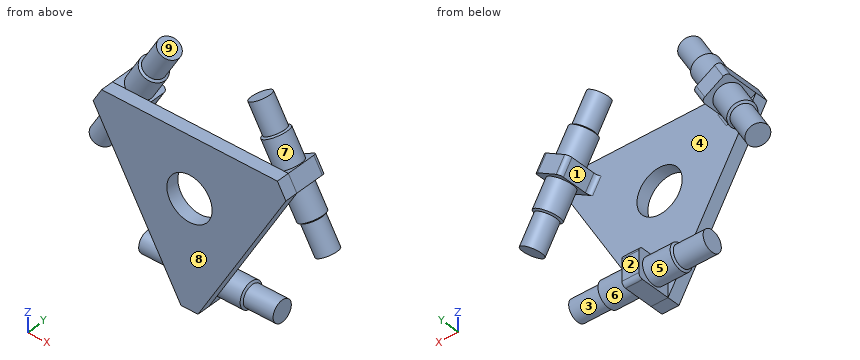
from build123d import *

# Parameters (mm, degrees)
BOSS_EXTRUDE1_DEPTH              = 3.81
F_17_32_0_53125_DIAMETER_HOLE1_D = 13.49375
BOSS_EXTRUDE2_DEPTH              = 10.16
CIRPATTERN19_COUNT               = 3
BOSS_EXTRUDE3_START              = -13.71
SKETCH6_R                        = 3.825
BOSS_EXTRUDE3_DEPTH              = 22.34
BOSS_EXTRUDE4_START              = -31.23
SKETCH7_R                        = 3.175
BOSS_EXTRUDE4_DEPTH              = 40.12
CIRPATTERN21_COUNT               = 3
CIRPATTERN28_COUNT               = 3
CHAMFER3_SIZE                    = 0.4
CHAMFER3_SIZE_2                  = 0.692820323
FILLET4_R                        = 1.27


with BuildPart() as part:
    # Sketch1 → Boss-Extrude1 (new body)
    with BuildSketch(Plane(origin=(0, 0, 0), x_dir=(1, 0, 0), z_dir=(0, 1, 0))):
        Polygon((2.54, 31.75), (-2.54, 31.75), (-28.76630657, -13.675295474), (-26.22630657, -18.074704526), (26.22630657, -18.074704526), (28.76630657, -13.675295474), align=None)
    extrude(amount=BOSS_EXTRUDE1_DEPTH)

    # 17/32 (0.53125) Diameter Hole1 (through all)
    with Locations(Plane(origin=(-6.6e-08, 3.81, -3.86e-07), x_dir=(0, 0, 1), z_dir=(0, 1, 0))):
        with Locations((0, 0)):
            Hole(F_17_32_0_53125_DIAMETER_HOLE1_D / 2)

    # Sketch5 → Boss-Extrude2 (add)
    with BuildSketch(Plane(origin=(0, 3.81, 0), x_dir=(1, 0, 0), z_dir=(0, 1, 0))):
        Polygon((-21.067340731, -9.230295474), (-28.76630657, -13.675295474), (-26.22630657, -18.074704526), (-18.527340731, -13.629704526), align=None)
    boss_extrude2 = extrude(amount=BOSS_EXTRUDE2_DEPTH)

    # CirPattern19: Boss-Extrude2 ×3 about axis
    cirpattern19_axis = Axis((0, 0, 0), (0, 1, 0))
    for i in range(1, CIRPATTERN19_COUNT):
        add(boss_extrude2.rotate(cirpattern19_axis, i * 360 / CIRPATTERN19_COUNT))

    # Sketch6 → Boss-Extrude3 (add)
    with BuildSketch(Plane(origin=(1.27, 0, 2.199704526), x_dir=(0.8660254037844383, 0, -0.5000000000000007), z_dir=(0.5000000000000007, 0, 0.8660254037844383)).offset(BOSS_EXTRUDE3_START)):
        with Locations((-27.305, 8.89)):
            Circle(SKETCH6_R)
    boss_extrude3 = extrude(amount=BOSS_EXTRUDE3_DEPTH)

    # Sketch7 → Boss-Extrude4 (add)
    with BuildSketch(Plane(origin=(5.585, 0, 9.67350376), x_dir=(0.8660254037844384, 0, -0.5000000000000007), z_dir=(0.5000000000000007, 0, 0.8660254037844384)).offset(BOSS_EXTRUDE4_START)):
        with Locations((-27.305, 8.89)):
            Circle(SKETCH7_R)
    boss_extrude4 = extrude(amount=BOSS_EXTRUDE4_DEPTH)

    # CirPattern21: Boss-Extrude3 ×3 about axis
    cirpattern21_axis = Axis((0, 0, 0), (0, 1, 0))
    for i in range(1, CIRPATTERN21_COUNT):
        add(boss_extrude3.rotate(cirpattern21_axis, i * 360 / CIRPATTERN21_COUNT))

    # CirPattern28: Boss-Extrude4 ×3 about axis
    cirpattern28_axis = Axis((0, 0, 0), (0, 1, 0))
    for i in range(1, CIRPATTERN28_COUNT):
        add(boss_extrude4.rotate(cirpattern28_axis, i * 360 / CIRPATTERN28_COUNT))

    # Chamfer3
    # the kernel refuses this chamfer: 0.692820323, 0.4 mm, written as the material it takes off along each edge
    with BuildSketch(Plane(origin=(-18.06182365, 8.89, 23.32600376), x_dir=(0.8660254037844383, 0, -0.5000000000000004), z_dir=(0, -1, 0))) as chamfer3_piece_1_section:
        Polygon((3.825, -CHAMFER3_SIZE), (3.825 - CHAMFER3_SIZE_2, 0), (3.825, 0), align=None)
    chamfer3_piece_1 = revolve(axis=Axis((-18.06182365, 8.89, 23.32600376), (0.5000000000000007, 0, 0.8660254037844383)), mode=Mode.PRIVATE)
    chamfer3_piece_1 = chamfer3_piece_1 - Plane(origin=(-18.164887991, 8.89, 23.147491086), x_dir=(0.8660254037844384, 0, -0.5000000000000007), z_dir=(-0.5000000000000007, 0, -0.8660254037844384)) * Cylinder(3.175, 16, mode=Mode.PRIVATE)
    add(chamfer3_piece_1, mode=Mode.SUBTRACT)
    with BuildSketch(Plane(origin=(-11.17, 8.89, -27.305), x_dir=(0, 0, 1), z_dir=(0, -1, 0))) as chamfer3_piece_2_section:
        Polygon((3.825, -CHAMFER3_SIZE), (3.825 - CHAMFER3_SIZE_2, 0), (3.825, 0), align=None)
    chamfer3_piece_2 = revolve(axis=Axis((-11.17, 8.89, -27.305), (-1, 0, 0)), mode=Mode.PRIVATE)
    chamfer3_piece_2 = chamfer3_piece_2 - Plane(origin=(-10.963871319, 8.89, -27.305), x_dir=(0, 0, 1), z_dir=(1, 0, 0)) * Cylinder(3.175, 16, mode=Mode.PRIVATE)
    add(chamfer3_piece_2, mode=Mode.SUBTRACT)
    with BuildSketch(Plane(origin=(11.17, 8.89, -27.305), x_dir=(0, 0, 1), z_dir=(0, -1, 0))) as chamfer3_piece_3_section:
        Polygon((3.825, CHAMFER3_SIZE), (3.825 - CHAMFER3_SIZE_2, 0), (3.825, 0), align=None)
    chamfer3_piece_3 = revolve(axis=Axis((11.17, 8.89, -27.305), (-1, 0, 0)), mode=Mode.PRIVATE)
    chamfer3_piece_3 = chamfer3_piece_3 - Plane(origin=(10.963871319, 8.89, -27.305), x_dir=(0, 0, 1), z_dir=(1, 0, 0)) * Cylinder(3.175, 16, mode=Mode.PRIVATE)
    add(chamfer3_piece_3, mode=Mode.SUBTRACT)
    with BuildSketch(Plane(origin=(29.23182365, 8.89, 3.97899624), x_dir=(-0.8660254037844392, 0, -0.49999999999999906), z_dir=(0, -1, 0))) as chamfer3_piece_4_section:
        Polygon((3.825, -CHAMFER3_SIZE), (3.825 - CHAMFER3_SIZE_2, 0), (3.825, 0), align=None)
    chamfer3_piece_4 = revolve(axis=Axis((29.23182365, 8.89, 3.97899624), (0.4999999999999995, 0, -0.8660254037844389)), mode=Mode.PRIVATE)
    chamfer3_piece_4 = chamfer3_piece_4 - Plane(origin=(29.12875931, 8.89, 4.157508914), x_dir=(-0.8660254037844389, 0, -0.49999999999999956), z_dir=(-0.49999999999999956, 0, 0.8660254037844389)) * Cylinder(3.175, 16, mode=Mode.PRIVATE)
    add(chamfer3_piece_4, mode=Mode.SUBTRACT)
    with BuildSketch(Plane(origin=(18.06182365, 8.89, 23.32600376), x_dir=(-0.8660254037844394, 0, -0.49999999999999895), z_dir=(0, -1, 0))) as chamfer3_piece_5_section:
        Polygon((3.825, CHAMFER3_SIZE), (3.825 - CHAMFER3_SIZE_2, 0), (3.825, 0), align=None)
    chamfer3_piece_5 = revolve(axis=Axis((18.06182365, 8.89, 23.32600376), (0.4999999999999995, 0, -0.8660254037844389)), mode=Mode.PRIVATE)
    chamfer3_piece_5 = chamfer3_piece_5 - Plane(origin=(18.164887991, 8.89, 23.147491086), x_dir=(-0.8660254037844389, 0, -0.49999999999999956), z_dir=(-0.49999999999999956, 0, 0.8660254037844389)) * Cylinder(3.175, 16, mode=Mode.PRIVATE)
    add(chamfer3_piece_5, mode=Mode.SUBTRACT)
    with BuildSketch(Plane(origin=(-29.23182365, 8.89, 3.97899624), x_dir=(0.8660254037844383, 0, -0.5000000000000004), z_dir=(0, -1, 0))) as chamfer3_piece_6_section:
        Polygon((3.825, CHAMFER3_SIZE), (3.825 - CHAMFER3_SIZE_2, 0), (3.825, 0), align=None)
    chamfer3_piece_6 = revolve(axis=Axis((-29.23182365, 8.89, 3.97899624), (0.5000000000000007, 0, 0.8660254037844383)), mode=Mode.PRIVATE)
    chamfer3_piece_6 = chamfer3_piece_6 - Plane(origin=(-29.12875931, 8.89, 4.157508914), x_dir=(0.8660254037844384, 0, -0.5000000000000007), z_dir=(-0.5000000000000007, 0, -0.8660254037844384)) * Cylinder(3.175, 16, mode=Mode.PRIVATE)
    add(chamfer3_piece_6, mode=Mode.SUBTRACT)

    # Fillet4
    fillet4_edges = [part.edges().sort_by_distance(p)[0] for p in [
        (-19.797340731, 3.81, 11.43),
        (-27.49630657, 13.97, 15.875),
        (-19.797340731, 13.97, 11.43),
        (19.797340731, 3.81, 11.43),
        (27.49630657, 13.97, 15.875),
        (19.797340731, 13.97, 11.43),
        (0, 3.81, -22.86),
        (0, 13.97, -31.75),
        (0, 13.97, -22.86),
    ]]
    fillet(fillet4_edges, radius=FILLET4_R)


solid = part.part
Part model, mm, in its own coordinate system. Face numbers are marked on the shaded views. A direction names the side the tool comes from. Give positions to 0.01 mm unless a question says otherwise; leave off trailing zeros. Loops run counter-clockwise (first coordinate to the right, second up) from the corner with the lowest first, then second, coordinate; pieces in that order, holes last. Notation, with made-up numbers: M -35,8.25 L 13,8.25 A11 ccw 13,23.25 Z; hole C -22,21.25 d7. An arc over 180 degrees is marked long. Put each result on its own line as item: value. Start each with the question number.
1) 3-axis set-ups, long thin cutter, end or side, ignore diameter. For the marked faces 1, 2, 3, 4 and 5: which of +Z, -Z, +X, -X, +Y, -Y reach the whole face in a straight line?
2) Saw through at C-C (y = 8.89). State how many separate pieces and enclosed holes the cut face has, then the cut area to 3 significant figures.
3) Flat gauge pins, fed straight in: pin 1 (8 mm diameter, centred on x = -21, z = 6.5, fed in from +Y); pin 2 (4 mm diameter, centred on x = 22, z = 6.5, fed in from +Y); pin 3 (4 mm diameter, centred on x = 2, y = 1, fed in from +Z); pin 4 (5 mm diameter, centred on x = -7.5, z = -13, fed in from +Y). Where does each tip first touch, or does it go through?
4) Saw through at D-D (z = -16.5). List the corners of the cut face in (x, y).
5) Probe probe 1 along Z at (x, y) = (0, 1.2); probe 2 along Y at (x, z) = (14, -6); probe 3 along Z at (x, y) = (0.5, 5.75). List the from-to ranges inside material, lowest first.
6) Pull direction Y, two halves, no side cores. Call the marked faces 6, 7, 8 and 9: +Y half, -Y half, draft (parallel to the pull), parting line (faces both ways), or undercut.
7) Saw through at B-B (x = 0). List the corners of the cut face in (y, z), then the cut area to 3 significant figures.
8) Saw through at A-A (y = 1.5). List the corners of the cut face in (x, z), then the cut area to 3 significant figures.
Numbers:
1. face 1: +Y
1. face 2: +Z, -Z, +X, -X, +Y
1. face 3: +X
1. face 4: none
1. face 5: -X
2. separate pieces: 3
2. enclosed holes: 0
2. area: 869 mm^2
3. pin 1: y = 13.97
3. pin 2: y = 11.26
3. pin 3: z = 18.07
3. pin 4: y = 3.81
4. outline: M -11.34,0 L 11.34,0 L 11.34,3.81 L -11.34,3.81 Z
5. probe 1: -31.75 to -6.75, 6.75 to 18.07
5. probe 2: 0 to 3.81
5. probe 3: -31.75 to -22.86
6. face 6: undercut
6. face 7: undercut
6. face 8: -Y half
6. face 9: draft
7. outline: M 0,-31.75 L 12.7,-31.75 A1.27 ccw 13.97,-30.48 L 13.97,-24.13 A1.27 ccw 12.7,-22.86 L 5.08,-22.86 A1.27 cw 3.81,-21.59 L 3.81,-6.75 L 0,-6.75 Z; M 0,6.75 L 3.81,6.75 L 3.81,18.07 L 0,18.07 Z
7. area: 228 mm^2
8. outline: M -28.77,13.68 L -2.54,-31.75 L 2.54,-31.75 L 28.77,13.68 L 26.23,18.07 L -26.23,18.07 Z; hole C 0,0 d13.49
8. area: 1,520 mm^2
